Input: dimensioned drawing with shaded views. Units: mm. Origin: part minimum x, y, z. A direction names the side the tool comes from. Give positions to 0.01 mm unless a question says otherwise; leave off trailing zeros. Write each loop counter-clockwise with the first axis right and the second up, starting at its lowest first coordinate (ties: lowest second). Pieces come first, ordered by that corner, then holes.
Q1. Section A-A (z = 16). Return the cut outline in (x, y).
Q2. Section D-D (y = 12). Return the cut outline in (x, z), plus the area to 3 significant figures.
Q3. Pin query (flat end, axial travel): pin 1 Ø1.5 at (x, z) = (3.5, 14) entering from +Y; pin 2 Ø2 at (y, z) = (27.5, 13) entering from +X; pin 3 Ø3 at (x, y) = (4.5, 9) entering from -Z; pin 4 Ø3.5 at (y, z) = (16, 16) entering from +X. Return the tip coordinate at first contact, or that it passes through.
Q4. Line query: line 1 (Z direction, x = 11, y = 16); line 2 (Z direction, x = 14.25, y = 16); line 3 (X direction, y = 25.5, z = 24). Output: solid intervals per line, ascending.
Q5. Mould query, pull axis Z, two halves, no side actions, for the marked faces 1, 2 and 3. Classes: +Z half, -Z half, draft (parallel to the pull), parting line (faces both ways), or undercut.
Q6. Reachability of the marked faces 4, 5 and 6 from +Z, -Z, +X, -X, +Y, -Y: full face, straight path, thin tool, end or side. Return the list, or none.
Q7. Section C-C (x = 12.5). Return the cut outline in (y, z), plus the area to 3 significant figures.
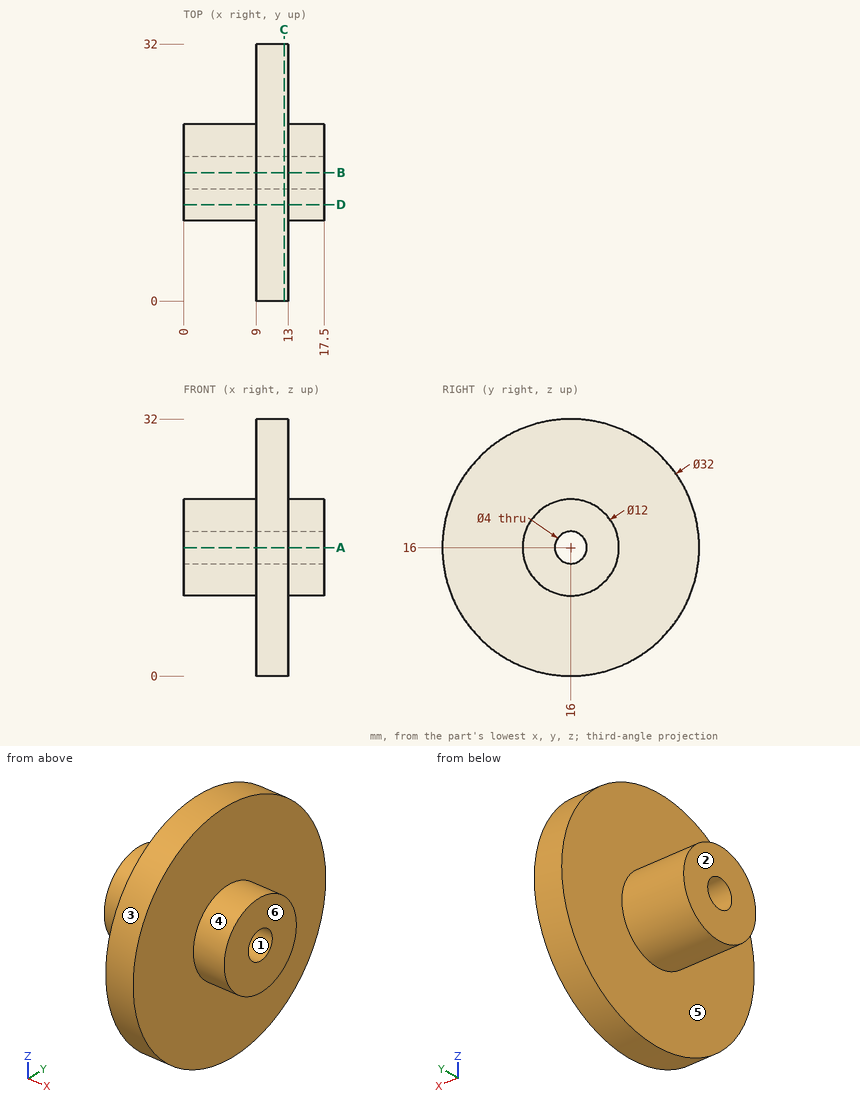
Computed:
1. outline: (0, 10) - (9, 10) - (9, 0) - (13, 0) - (13, 10) - (17.5, 10) - (17.5, 14) - (0, 14) - close; (0, 18) - (17.5, 18) - (17.5, 22) - (13, 22) - (13, 32) - (9, 32) - (9, 22) - (0, 22) - close
2. outline: (0, 11.53) - (9, 11.53) - (9, 0.51) - (13, 0.51) - (13, 11.53) - (17.5, 11.53) - (17.5, 20.47) - (13, 20.47) - (13, 31.49) - (9, 31.49) - (9, 20.47) - (0, 20.47) - close
2. area: 245 mm2
3. pin 1: stops at y = 21.87
3. pin 2: stops at x = 13
3. pin 3: stops at z = 13.6
3. pin 4: passes through
4. line 1: z = 0 to 14, 18 to 32
4. line 2: z = 10 to 14, 18 to 22
4. line 3: x = 9 to 13
5. face 1: undercut
5. face 2: draft
5. face 3: parting line
6. face 4: +X
6. face 5: -X
6. face 6: +Z, -Z, +X, +Y, -Y
7. outline: circle Ø32 at (16, 16); hole circle Ø4 at (16, 16)
7. area: 792 mm2
